from build123d import *

# Parameters (mm, degrees)
SKETCH1_W           = 6.35
SKETCH1_H           = 6.35
BOSS_EXTRUDE1_DEPTH = 39.6875
SKETCH4_W           = 11.064537346
SKETCH4_H           = 8.106256658
SKETCH4_R           = 3.175
CUT_EXTRUDE3_DEPTH  = 3.175
CUT_EXTRUDE4_START  = -20.515625
SKETCH5_W           = 9.216364604
SKETCH5_H           = 9.38217528
SKETCH5_R           = 3.429
CUT_EXTRUDE4_DEPTH  = 20.515625


with BuildPart() as part:
    # Sketch1 → Boss-Extrude1 (new body)
    with BuildSketch(Plane(origin=(0, 0, 0), x_dir=(0, 0, -1), z_dir=(1, 0, 0))):
        Rectangle(SKETCH1_W, SKETCH1_H)
    extrude(amount=BOSS_EXTRUDE1_DEPTH)

    # Sketch4 → Cut-Extrude3 (cut)
    with BuildSketch(Plane.ZY):
        Rectangle(SKETCH4_W, SKETCH4_H)
        Circle(SKETCH4_R, mode=Mode.SUBTRACT)
    extrude(amount=-CUT_EXTRUDE3_DEPTH, mode=Mode.SUBTRACT)

    # Sketch5 → Cut-Extrude4 (cut)
    with BuildSketch(Plane.ZY.offset(-3.175).offset(CUT_EXTRUDE4_START)):
        Rectangle(SKETCH5_W, SKETCH5_H)
        Circle(SKETCH5_R, mode=Mode.SUBTRACT)
    extrude(amount=CUT_EXTRUDE4_DEPTH, mode=Mode.SUBTRACT)


solid = part.part
The model under review builds one solid part; all positions refer to its coordinate system, in mm. A direction names the side the tool comes from. Round coordinates to 2 decimals unless told otherwise and drop trailing zeros. Loops run counter-clockwise (first coordinate to the right, second up) from the corner with the lowest first, then second, coordinate; pieces in that order, holes last. Notation, with made-up numbers: M 4.5,-19 L 38.5,-19 A33 cw 38.5,13 Z; hole C 61,42 d11. An arc over 180 degrees is marked long. Answer as CSV lines item,"result". Start each with the question number.
Item 1: For faces 1 (the face through (1.57, -3.1, -0.69)), 2 (the face through (23.691, 3, -3)), 3 (the face through (13.58, -2.44, 2.41)), 4 (the face through (13.58, 2.41, 2.44)), 5 (the face through (13.58, -2.41, -2.44)), list the 3-axis set-ups (+Z, -Z, +X, -X, +Y, -Y) from which the entire face can be reached by the end or side of a thin tool; tool diameter is ignored.
Item 2: Wall thickness on line 1 (Z direction, x = 6, y = -2); line 2 (Y direction, x = 6.5, z = 2.75); line 3 (Y direction, x = 3, z = 2): over which ranges is each line inside the solid? List them lowest first. Write a range as [from, to].
Item 3: Insertion check: P1, Ø1, axis at y = -2.5, z = 0.5, coming from the -X side; P2, Ø1.5, axis at x = 15.5, y = -2.5, coming from the +Z side. Each pin has a flat end and moves straight along its axis. Give the tip position at first contact, or say it passes through.
Item 4: Consider section A-A (x = 4.5). Write out the cut boundary in (y, z) (3 decimals), then the cut area to 3 significant figures.
Answer:
1,face 1,"-X"
1,face 2,"-Z, -X, +Y"
1,face 3,"+Z, -X, -Y"
1,face 4,"+Z, -X, +Y"
1,face 5,"-Z, -X, -Y"
2,line 1,"z = [-2.79, 2.79]"
2,line 2,"y = [-2.05, 2.05]"
2,line 3,"y = [-2.47, 2.47]"
3,P1,"stops at x = 0"
3,P2,"stops at z = 2.95"
4,outline,"M -3.175,-1.295 A3.429 ccw -1.295,-3.175 L 1.295,-3.175 A3.429 ccw 3.175,-1.295 L 3.175,1.295 A3.429 ccw 1.295,3.175 L -1.295,3.175 A3.429 ccw -3.175,1.295 Z"
4,area,"35.2 mm^2"
